Can you work these out from the model? Positions are in its coordinate system, mm. Face numbers are marked on the shaded views. Give positions to 0.01 mm unless a question says otherwise; leave off trailing zeros. Write each loop counter-clockwise with the first axis right and the second up, starting at its lowest first coordinate (ties: lowest second). Pieces come first, ordered by that corner, then holes. Notation, with made-up numbers: (8, 35.5) - (43, 35.5) arc R15 ccw to (43, 57.5) - close; hole circle Ø8 at (-12.75, 58.25). An arc over 180 degrees is marked (long way). Return JSON: item names as keys, results as strings. Group by question number.
from build123d import *

# Parameters (mm, degrees)
BOSS_EXTRUDE1_DEPTH = 38.1
SKETCH2_R           = 7.9375
CUT_EXTRUDE1_DEPTH  = 38.1


with BuildPart() as part:
    # Sketch1 → Boss-Extrude1 (new body)
    with BuildSketch(Plane.XY):
        Polygon((0, 0), (0, 12.7), (38.1, 2.54), (38.1, 0), align=None)
    extrude(amount=BOSS_EXTRUDE1_DEPTH)

    # Sketch2 → Cut-Extrude1 (cut)
    with BuildSketch(Plane.XZ):
        with Locations((19.05, 19.05)):
            Circle(SKETCH2_R)
    extrude(amount=-CUT_EXTRUDE1_DEPTH, mode=Mode.SUBTRACT)


solid = part.part
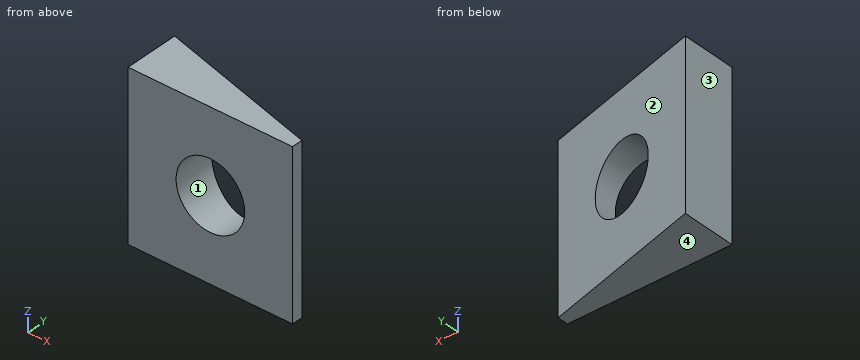
1) Imagine slicing it at A-A, the plane x = 19.05. Write out the boundary of the cut face in (y, z).
2) Imagine slicing it at B-B, the plane z = 19.05. Write out the boundary of the cut face in (x, y).
3) Imagine slicing it at D-D, the plane z = 9.5. Write out the boundary of the cut face in (x, y), and give its area (3 significant figures).
4) I need wall thicknesses on line 1 along Z through (x, y) = (19.05, 5); line 2 along X through (y, z) = (6.75, 19.05); line 3 along Y through (x, z) = (12.5, 2). Which ranges of each line are inside material? Lowest first, please.
5) We'd pull the mould along X, two halves only. Please class the marked faces 1, 2, 3 and 4: pulls with the +X half, pulls with the -X half, needs draft (parallel to the pull), parting line crosses it, or undercut.
6) Will this pin go through, and if not, where does the flat tip stop? pin 1 Ø1 at (x, z) = (21.5, 14) entering from -Y.
Resolved:
{
 "1": {"outline": "(0, 0) - (7.62, 0) - (7.62, 11.11) - (0, 11.11) - close; (0, 26.99) - (7.62, 26.99) - (7.62, 38.1) - (0, 38.1) - close"},
 "2": {"outline": "(0, 0) - (11.11, 0) - (11.11, 9.74) - (0, 12.7) - close; (26.99, 0) - (38.1, 0) - (38.1, 2.54) - (26.99, 5.5) - close"},
 "3": {"outline": "(0, 0) - (38.1, 0) - (38.1, 2.54) - (0, 12.7) - close", "area": "290 mm^2"},
 "4": {"line 1": "0 to 11.11, 26.99 to 38.1", "line 2": "0 to 11.11", "line 3": "0 to 9.37"},
 "5": {"face 1": "undercut", "face 2": "pulls with the +X half", "face 3": "pulls with the -X half", "face 4": "needs draft"},
 "6": {"pin 1": "through"}
}
